```python
from build123d import *

# Parameters (mm, degrees)
SKETCH1_W           = 30
SKETCH1_H           = 11
SKETCH1_W_2         = 22
SKETCH1_H_2         = 6
BOSS_EXTRUDE1_DEPTH = 1.5
SKETCH2_R           = 1
CUT_EXTRUDE1_DEPTH  = 5
SKETCH3_R           = 9
BOSS_EXTRUDE2_DEPTH = 27
SKETCH5_W           = 28
SKETCH5_H           = 21
BOSS_EXTRUDE3_DEPTH = 3
SKETCH6_R           = 1.5
BOSS_EXTRUDE4_DEPTH = 8
SKETCH7_R           = 1.5
SKETCH7_W           = 16.5
SKETCH7_H           = 16.5
BOSS_EXTRUDE5_DEPTH = 4


with BuildPart() as part:
    # Sketch1 → Boss-Extrude1 (new body)
    with BuildSketch(Plane.XY):
        Polygon((32, 0), (32, 20), (15, 23), (-15, 23), (-32, 20), (-32, 0), align=None)
        with Locations((0, 28.5)):
            Rectangle(SKETCH1_W, SKETCH1_H)
        with Locations((0, 37)):
            Rectangle(SKETCH1_W_2, SKETCH1_H_2)
    extrude(amount=BOSS_EXTRUDE1_DEPTH)

    # Sketch2 → Cut-Extrude1 (cut)
    with BuildSketch(Plane.XY.offset(1.5)):
        with Locations((20, 3)):
            Circle(SKETCH2_R)
        with Locations((0, 3)):
            Circle(SKETCH2_R)
        with Locations((-20, 3)):
            Circle(SKETCH2_R)
        with Locations((-30, 15)):
            Circle(SKETCH2_R)
        with Locations((30, 15)):
            Circle(SKETCH2_R)
    extrude(amount=-CUT_EXTRUDE1_DEPTH, mode=Mode.SUBTRACT)

    # Sketch3 → Boss-Extrude2 (add)
    with BuildSketch(Plane.XY.offset(1.5)):
        with Locations((0, 30.5)):
            Circle(SKETCH3_R)
    extrude(amount=BOSS_EXTRUDE2_DEPTH)

    # Sketch5 → Boss-Extrude3 (add)
    with BuildSketch(Plane(origin=(0, 0, 0), x_dir=(-1, 0, 0), z_dir=(0, 0, -1))):
        with Locations((-1, 17.5)):
            Rectangle(SKETCH5_W, SKETCH5_H)
    extrude(amount=BOSS_EXTRUDE3_DEPTH)

    # Sketch6 → Boss-Extrude4 (add)
    with BuildSketch(Plane.XY.offset(1.5)):
        with Locations((22, 18)):
            Circle(SKETCH6_R)
        with Locations((-22, 18)):
            Circle(SKETCH6_R)
    extrude(amount=BOSS_EXTRUDE4_DEPTH)

    # Sketch7 → Boss-Extrude5 (add)
    with BuildSketch(Plane.XY.offset(1.5)):
        with Locations((-8.75, 31)):
            Circle(SKETCH7_R)
        with Locations((8.75, 31)):
            Circle(SKETCH7_R)
        with Locations((0, 31)):
            Rectangle(SKETCH7_W, SKETCH7_H)
    extrude(amount=BOSS_EXTRUDE5_DEPTH)


solid = part.part
```
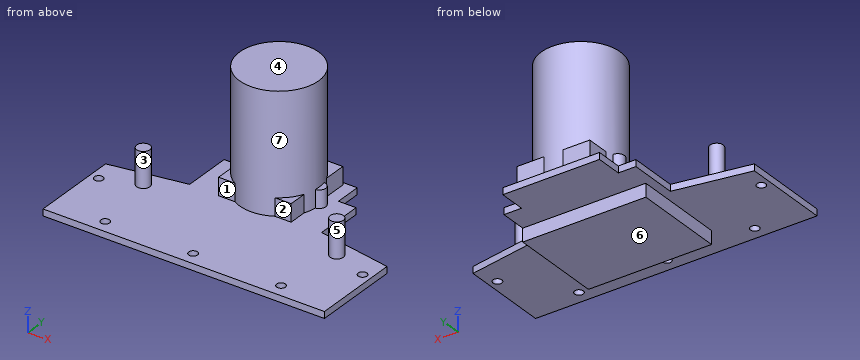
Input: part model. Units: mm. Frame: model coordinates. Face numbers are marked on the shaded views. A direction names the side the tool comes from. Coordinates: 2 decimals unless noted, no trailing zeros. Write each loop counter-clockwise with the first axis right and the second up, starting at its lowest first coordinate (ties: lowest second). Pieces come first, ordered by that corner, then holes.
1) Section A-A on y = 10. Output: boundary loops of the cut face in (x, z), and give its area (3 significant figures).
2) Pin query (flat end, axial travel): pin 1 Ø8 at (x, y) = (11.5, 32) entering from +Z; pin 2 Ø1.5 at (x, y) = (-22, 18) entering from +Z; pin 3 Ø0.8 at (y, z) = (38, 0.5) entering from +X; pin 4 Ø3 at (x, z) = (-19.5, 2.5) entering from +Y. Return the tip coordinate at first contact, or that it passes through.
3) Section C-C on z = 25. Output: boundary loops of the cut face in (x, y), and give its area (3 significant figures).
4) Mould query, pull axis X, two halves, no side actions, for the marked faces 5, 6 and 7. Classes: pulls with the +X half, pulls with the -X half, needs draft (parallel to the pull), parting line crosses it, or undercut.
5) Material intervals for line 1 along Z through (x, y) = (-11, 33); line 2 along Y through (x, z) = (-20, 0.55); line 3 along Z through (x, y) = (-4, 38.5), sorted ascending.
6) Section D-D on x = -14. Output: boundary loops of the cut face in (y, z), and give its area (3 significant figures).
7) Set-up query: the marked faces 1, 2, 3 and 4. Return all of +Z, -Z, +X, -X, +Y, -Y with unobstructed straight access to the full face (end or side cutting, diameter ignored); none if empty.
8) Section B-B on x = -30. Output: boundary loops of the cut face in (y, z).
Check result:
1. outline: (-32, 0) - (-13, 0) - (-13, -3) - (15, -3) - (15, 0) - (32, 0) - (32, 1.5) - (-32, 1.5) - close
1. area: 180 mm2
2. pin 1: stops at z = 28.5
2. pin 2: stops at z = 9.5
2. pin 3: stops at x = 11
2. pin 4: stops at y = 22.4
3. outline: circle Ø18 at (0, 30.5)
3. area: 254 mm2
4. face 5: undercut
4. face 6: needs draft
4. face 7: parting line crosses it
5. line 1: z = 0 to 1.5
5. line 2: y = 0 to 2, 4 to 22.12
5. line 3: z = 0 to 28.5
6. outline: (0, 0) - (34, 0) - (34, 1.5) - (0, 1.5) - close
6. area: 51.0 mm2
7. face 1: +Z, -X, -Y
7. face 2: +Z, +X, -Y
7. face 3: +Z
7. face 4: +Z, +X, -X, +Y, -Y
8. outline: (0, 0) - (14, 0) - (14, 1.5) - (0, 1.5) - close; (16, 0) - (20.35, 0) - (20.35, 1.5) - (16, 1.5) - close
